from build123d import *

# Parameters (mm, degrees)
SKETCH2_R                = 15.875
BOSS_EXTRUDE1_DEPTH      = 8.89
SKETCH3_R                = 13.97
BOSS_EXTRUDE2_DEPTH      = 0.3175
SKETCH4_R                = 14.0462
BOSS_EXTRUDE3_DEPTH      = 0.3175
CUT_EXTRUDE2_DEPTH       = 10.525
SKETCH7_R                = 11.43
SKETCH7_R_2              = 9.525
CUT_EXTRUDE3_DEPTH       = 0.3175
SKETCH9_R                = 4.7625
BOSS_EXTRUDE4_DEPTH      = 25.4
BOSS_EXTRUDE4_DEPTH_BACK = 0.254


with BuildPart() as part:
    # Sketch2 → Boss-Extrude1 (new body)
    with BuildSketch(Plane(origin=(0, 0, 0), x_dir=(1, 0, 0), z_dir=(0, 1, 0))):
        Circle(SKETCH2_R)
    extrude(amount=BOSS_EXTRUDE1_DEPTH)

    # Sketch3 → Boss-Extrude2 (add)
    with BuildSketch(Plane(origin=(0, 8.89, 0), x_dir=(1, 0, 0), z_dir=(0, 1, 0))):
        Circle(SKETCH3_R)
    extrude(amount=BOSS_EXTRUDE2_DEPTH)

    # Sketch4 → Boss-Extrude3 (add)
    with BuildSketch(Plane(origin=(0, 0, 0), x_dir=(-1, 0, 0), z_dir=(0, -1, 0))):
        Circle(SKETCH4_R)
    extrude(amount=BOSS_EXTRUDE3_DEPTH)

    # Sketch5 → Cut-Extrude2 (cut, through all)
    with BuildSketch(Plane(origin=(0, -0.3175, 0), x_dir=(-1, 0, 0), z_dir=(0, -1, 0))):
        with BuildLine():
            ThreePointArc((15.875, 0), (3.303921778, 15.527386319), (-14.499768616, 6.463152102))
            ThreePointArc((-14.499768616, 6.463152102), (-12.112281343, 8.677516697), (-9.382547241, 10.452920248))
            ThreePointArc((-9.382547241, 10.452920248), (5.723049859, 12.827409511), (14.0462, 0))
            ThreePointArc((14.0462, 0), (5.723049859, -12.827409511), (-9.382547241, -10.452920248))
            ThreePointArc((-9.382547241, -10.452920248), (-12.112281343, -8.677516697), (-14.499768616, -6.463152102))
            ThreePointArc((-14.499768616, -6.463152102), (3.303921778, -15.527386319), (15.875, 0))
        make_face()
        with BuildLine():
            ThreePointArc((14.0462, 0), (5.723049859, 12.827409511), (-9.382547241, 10.452920248))
            ThreePointArc((-9.382547241, 10.452920248), (-4.835884527, 12.180274323), (0, 12.7))
            ThreePointArc((0, 12.7), (8.980256121, 8.980256121), (12.7, 0))
            ThreePointArc((12.7, 0), (8.980256121, -8.980256121), (0, -12.7))
            ThreePointArc((0, -12.7), (-4.835884527, -12.180274323), (-9.382547241, -10.452920248))
            ThreePointArc((-9.382547241, -10.452920248), (5.723049859, -12.827409511), (14.0462, 0))
        make_face()
    extrude(amount=-CUT_EXTRUDE2_DEPTH, mode=Mode.SUBTRACT)

    # Sketch6 → Cut-Revolve1 (revolve, cut)
    with BuildSketch(Plane(origin=(0, 0, 0), x_dir=(0, 0, -1), z_dir=(1, 0, 0))):
        with BuildLine():
            Line((0, -5.08), (0, 0))
            Line((0, 0), (0, 4.445))
            Line((0, 4.445), (0, 13.97))
            ThreePointArc((0, 13.97), (-9.525, 4.445), (0, -5.08))
        make_face()
    revolve(axis=Axis((0, -5.08, 0), (0, 1, 0)), mode=Mode.SUBTRACT)

    # Sketch7 → Cut-Extrude3 (cut)
    with BuildSketch(Plane(origin=(0, 9.2075, 0), x_dir=(1, 0, 0), z_dir=(0, 1, 0))):
        Circle(SKETCH7_R)
        Circle(SKETCH7_R_2, mode=Mode.SUBTRACT)
    extrude(amount=-CUT_EXTRUDE3_DEPTH, mode=Mode.SUBTRACT)

    # Sketch9 → Boss-Extrude4 (add, two sides)
    with BuildSketch(Plane(origin=(15.24, 0, 0), x_dir=(0, 0, -1), z_dir=(1, 0, 0))) as boss_extrude4_sk:
        with Locations((0, 4.445)):
            Circle(SKETCH9_R)
    extrude(amount=BOSS_EXTRUDE4_DEPTH)
    extrude(boss_extrude4_sk.sketch, amount=-BOSS_EXTRUDE4_DEPTH_BACK)

    # Sketch11 → Cut-Revolve2 (revolve, cut)
    with BuildSketch(Plane.XY):
        Polygon((40.64, -0.3175), (40.64, 0.3175), (40.005, -0.3175), align=None)
    revolve(axis=Axis((40.64, 4.445, 0), (-1, 0, 0)), mode=Mode.SUBTRACT)


solid = part.part
Model file for the job. Use its own axes, mm. A direction names the side the tool comes from. Give positions to 0.01 mm unless a question says otherwise; leave off trailing zeros. Loops run counter-clockwise (first coordinate to the right, second up) from the corner with the lowest first, then second, coordinate; pieces in that order, holes last. Notation, with made-up numbers: (61, 70.25) - (100, 70.25) arc R37 ccw to (100, 106.25) - close; hole circle Ø9 at (39, 60.25). An arc over 180 degrees is marked (long way). Use one line per item in the form item = value.
(1) 3-axis set-ups, long thin cutter, end or side, ignore diameter. For faces 4 (the face through (10.902, 9.051, -3.433)), 5 (the face through (11.44, 9.208, -1.94)), 6 (the face through (40.64, 5, 0)), 7 (the face through (14.2, 0, -0.8)), 8 (the face through (15, 4.4, 5.2)): which of +Z, -Z, +X, -X, +Y, -Y reach the whole face in a straight line?
Determined:
face_4 = +Y
face_5 = +Z, -Z, +X, -X, +Y
face_6 = +Z, -Z, +X, +Y, -Y
face_7 = -Y
face_8 = +Z, +X
(2) Drill centre lines: L1, parallel to X at y = 2, z = -7.75; L2, parallel to X at y = 1, z = 4.5; L3, parallel to Z at x = 5, y = 4.5. Where is each one in solid material? Low to high.
Determined:
L1 = -10.06 to -4.97, 4.97 to 13.21
L2 = -11.88 to -7.66, 7.66 to 15.22
L3 = -12.14 to -8.11, 8.11 to 12.14
(3) Drop flat-ended pins along their axis: P1, Ø1.5, axis at x = 21, y = 5, coming from the -Z side; P2, Ø2, axis at y = 5.5, z = 5.5, coming from the -X side; P3, Ø5, axis at x = 13.5, y = 4.5, coming from the -Z side. Give the stop position or say it passes through.
Determined:
P1 = -4.76
P2 = -11.88
P3 = -9.48
(4) Cut at D-D (x = 19). Give the cut face in (y, z) (1 decimal), then the cut area to 3 significant figures.
Determined:
outline = circle Ø9.5 at (4.4, 0)
area = 71.3 mm^2
(5) Pull direction X, two halves, no side cores. Call faces 1 (the face through (15, 4.4, -5.2)), 2 (the face through (14.2, 8.89, -0.8)), 3 (the face through (7, -0.318, -6)): pulls with the +X half, pulls with the -X half, needs draft (parallel to the pull), parting line crosses it, or undercut.
Determined:
face_1 = pulls with the +X half
face_2 = undercut
face_3 = needs draft
